Read the model definition and answer for the solid it produces. Units are mm, in the model's axes. A direction names the side the tool comes from. Round coordinates to 2 decimals unless told otherwise and drop trailing zeros. Write each loop counter-clockwise with the first axis right and the second up, starting at its lowest first coordinate (ties: lowest second). Pieces come first, ordered by that corner, then holes. Notation, with made-up numbers: (-14.5, 56.5) - (43.5, 56.5) arc R17 cw to (43.5, 68.5) - close; hole circle Ø9 at (-38, -2). An arc over 180 degrees is marked (long way). Use one line per item in the form item = value. Start each with the question number.
1) The part is cut by section C-C, the plane z = 1. Give the vertices of the cut face in (x, y), plus the area to 3 significant figures.
2) The part is cut by section D-D, the plane y = 0. Give the vertices of the cut face in (x, z), plus the area to 3 significant figures.
3) For a pull along X with two mould halves and no side action, classify faces 4 (the face through (2, -2, 35)), 5 (the face through (-0.4, 0, 38)), 6 (the face through (-1.08, -4.88, 36.97)), 7 (the face through (0, 0, 37.8)) as released by +X, released by -X, zero draft, split by the parting line, or undercut.
4) Each of these flat-tipped pins is pushed along its axis until it touches: pin 1 (4 mm diameter, centred on y = 2, z = 6.5, fed in from +X); pin 2 (1.5 mm diameter, centred on x = 0, z = 21.5, fed in from +Y); pin 3 (4 mm diameter, centred on y = 0.5, z = 8.5, fed in from -X). Where does it stop, or does it pass through?
5) Consider line 1 along Z through (x, y) = (-2.5, -3.75); line 2 along Z through (x, y) = (0, 1.5); line 3 along Y through (x, z) = (0, 5). Determine where each line is inside the solid, lowest interval first. Write a range as from..to.
6) The part is cut by section B-B, the plane x = 0. Give the vertices of the cut face in (y, z), plus the area to 3 significant figures.
7) The part is cut by section A-A, the plane y = 3. Give the vertices of the cut face in (x, z), plus the area to 3 significant figures.
8) For faces 1 (the face through (-0.54, -2.44, 14.72)), 2 (the face through (0.4, 0, 38)), 3 (the face through (0, 0, -5)), determine the directions among +Z, -Z, +X, -X, +Y, -Y from which every point of the face is accessible in a straight line to the end or side of a thin tool.
from build123d import *

# Parameters (mm, degrees)
EXTRUDE_1_DEPTH      = 35
EXTRUDE_1_DEPTH_BACK = 5
SKETCH_1_R           = 2.5
SKETCH_2_R           = 5
EXTRUDE_2_DEPTH      = 4
SKETCH_3_W           = 0.8
SKETCH_3_H           = 11.021006482
CUT_EXTRUDE_1_DEPTH  = 1.2


with BuildPart() as part:
    # Эскиз1 → Вытянуть1 (new, two sides: drawn at the far end of the back side and taken through both)
    with BuildSketch(Plane.XY.offset(-EXTRUDE_1_DEPTH_BACK)):
        Circle(SKETCH_1_R)
    extrude(amount=EXTRUDE_1_DEPTH + EXTRUDE_1_DEPTH_BACK)

    # Эскиз2 → Вытянуть2 (add)
    with BuildSketch(Plane.XY.offset(35)):
        Circle(SKETCH_2_R)
    extrude(amount=EXTRUDE_2_DEPTH)

    # Эскиз3 → Вырез-Вытянуть1 (cut)
    with BuildSketch(Plane.XY.offset(39)):
        with Locations((0, 0.044379892)):
            Rectangle(SKETCH_3_W, SKETCH_3_H)
    extrude(amount=-CUT_EXTRUDE_1_DEPTH, mode=Mode.SUBTRACT)


solid = part.part
Geometry results:
q1.outline = circle Ø5 at (0, 0)
q1.area = 19.6 mm2
q2.outline = (-5, 35) - (-2.5, 35) - (-2.5, -5) - (2.5, -5) - (2.5, 35) - (5, 35) - (5, 39) - (0.4, 39) - (0.4, 37.8) - (-0.4, 37.8) - (-0.4, 39) - (-5, 39) - close
q2.area = 239 mm2
q3.face_4 = zero draft
q3.face_5 = undercut
q3.face_6 = split by the parting line
q3.face_7 = undercut
q4.pin_1 = 2.5
q4.pin_2 = 2.5
q4.pin_3 = -2.5
q5.line_1 = 35..39
q5.line_2 = -5..37.8
q5.line_3 = -2.5..2.5
q6.outline = (-5, 35) - (-2.5, 35) - (-2.5, -5) - (2.5, -5) - (2.5, 35) - (5, 35) - (5, 37.8) - (-5, 37.8) - close
q6.area = 228 mm2
q7.outline = (-4, 35) - (4, 35) - (4, 39) - (0.4, 39) - (0.4, 37.8) - (-0.4, 37.8) - (-0.4, 39) - (-4, 39) - close
q7.area = 31.0 mm2
q8.face_1 = -Z
q8.face_2 = +Z, +Y, -Y
q8.face_3 = -Z, +X, -X, +Y, -Y
